Autodesk Inventor part; units mm, degrees
ref_plane "YZ Plane" through (0, 0, 0) normal (1, 0, 0) x (0, 1, 0)
ref_plane "XZ Plane" through (0, 0, 0) normal (0, 1, 0) x (-1, 0, 0)
ref_plane "XY Plane" through (0, 0, 0) normal (0, 0, 1) x (1, 0, 0)
sketch "スケッチ1" plane through (0, 0, 0) normal (0, 0, 1) x (1, 0, 0)
  line L0 (-12.5, -12.5) -> (12.5, -12.5) construction
  line L1 (12.5, -12.5) -> (12.5, 12.5) construction
  line L2 (12.5, 12.5) -> (-12.5, 12.5) construction
  line L3 (-12.5, 12.5) -> (-12.5, -12.5) construction
  line L4 (-12.5, -12.5) -> (12.5, 12.5) construction
  line L5 (12.5, -12.5) -> (-12.5, 12.5) construction
  line L6 (-8.1, 12.5) -> (-12.5, 12.5)
  line L7 (-12.5, 12.5) -> (-12.5, 8.1)
  line L8 (8.1, 12.5) -> (12.5, 12.5)
  line L9 (12.5, 12.5) -> (12.5, 8.1)
  line L10 (-12.5, -8.1) -> (-12.5, -12.5)
  line L11 (-12.5, -12.5) -> (-8.1, -12.5)
  line L12 (8.1, -12.5) -> (12.5, -12.5)
  line L13 (12.5, -12.5) -> (12.5, -8.1)
  line L14 (-6, 12.5) -> (-6, 14.5)
  line L15 (-6, 14.5) -> (6, 14.5)
  line L16 (6, 14.5) -> (6, 12.5)
  arc A0 (-8.1, 12.5) -> (-6, 12.5) centre (-7.05, 12.5) ccw
  arc A1 (6, 12.5) -> (8.1, 12.5) centre (7.05, 12.5) ccw
  line L17 (0, 12.5) -> (0, 0) construction
  line L18 (0, 0) -> (12.5, 0) construction
  line L19 (-12.5, 6) -> (-14.5, 6) construction
  line L20 (-14.5, 6) -> (-14.5, -6) construction
  line L21 (-14.5, -6) -> (-12.5, -6) construction
  arc A2 (-12.5, 6) -> (-12.5, 8.1) centre (-12.5, 7.05) ccw
  arc A3 (-12.5, -8.1) -> (-12.5, -6) centre (-12.5, -7.05) ccw construction
  line L22 (-6, -12.5) -> (-6, -14.5)
  line L23 (-6, -14.5) -> (6, -14.5)
  line L24 (6, -14.5) -> (6, -12.5)
  arc A4 (-6, -12.5) -> (-8.1, -12.5) centre (-7.05, -12.5) ccw
  arc A5 (8.1, -12.5) -> (6, -12.5) centre (7.05, -12.5) ccw
  line L25 (12.5, 6) -> (14.5, 6) construction
  line L26 (14.5, 6) -> (14.5, -6) construction
  line L27 (14.5, -6) -> (12.5, -6) construction
  arc A6 (12.5, 8.1) -> (12.5, 6) centre (12.5, 7.05) ccw construction
  arc A7 (12.5, -6) -> (12.5, -8.1) centre (12.5, -7.05) ccw construction
  line L28 (-9.05, 12.5) -> (-5.95, 12.5) construction
  line L29 (-5.95, 12.5) -> (-5.95, 9.5) construction
  line L30 (-5.95, 9.5) -> (-9.05, 9.5) construction
  line L31 (-9.05, 9.5) -> (-9.05, 12.5) construction
  line L32 (-12.5, 9.05) -> (-9.5, 9.05) construction
  line L33 (-9.5, 9.05) -> (-9.5, 5.95) construction
  line L34 (-9.5, 5.95) -> (-12.5, 5.95) construction
  line L35 (-12.5, 5.95) -> (-12.5, 9.05) construction
  line L36 (-6.7322, 8.5) -> (6.7322, 8.5)
  line L37 (6.7322, 8.5) -> (0, 1.7678)
  line L38 (0, 1.7678) -> (-6.7322, 8.5)
  line L39 (-8.5, 6.7322) -> (-8.5, -6.7322)
  line L40 (-8.5, -6.7322) -> (-1.7678, 0)
  line L41 (-1.7678, 0) -> (-8.5, 6.7322)
  line L42 (-6.7322, -8.5) -> (6.7322, -8.5)
  line L43 (6.7322, -8.5) -> (0, -1.7678)
  line L44 (0, -1.7678) -> (-6.7322, -8.5)
  line L45 (8.5, 6.7322) -> (8.5, -6.7322)
  line L46 (8.5, -6.7322) -> (1.7678, 0)
  line L47 (1.7678, 0) -> (8.5, 6.7322)
  line L48 (-7.5, 12.5) -> (-7.5, 9.5) construction
  line L49 (-9.5, 7.5) -> (-12.5, 7.5) construction
  line L50 (-12.5, -12.5) -> (-12.5, 12.5)
  line L51 (12.5, -12.5) -> (12.5, 12.5)
  dimension "d0" = 25
  dimension "d1" = 1.05
  dimension "d2" = 2
  dimension "d3" = 6.5
  dimension "d4" = 3.1
  dimension "d6" = 3
  dimension "d8" = 3
  dimension "d9" = 2.5
  dimension "d10" = 2.5
  dimension "d11" = 2.5
  dimension "d12" = 2.5
  dimension "d13" = 4
  dimension "d17" = 5
  dimension "d18" = 5
  dimension "d31" = 25
extrude "押し出し1" add sketch "スケッチ1" along normal blind 2.5
mirror "ミラー1" about plane through (0, 0, 0) normal (0, 0, -1) of "押し出し1"
sketch "スケッチ2" plane through (-12.5, -12.5, 2.5) normal (0, -1, 0) x (1, 0, 0)
  line L0 (0, -5) -> (0, 0)
  line L1 (6.5, 0) -> (18.5, 0) construction
  line L2 (12.5, 0) -> (12.5, -5) construction
  point P0 (12.5, -2.5)
  point P1 (2.7, -2.5)
  point P2 (22.3, -2.5)
  point P3 (0, -2.5)
  dimension "d19" = 2.7
hole "穴1" at (-9.8, -12.5, 0) at (9.8, -12.5, 0) direction (0, 1, 0) diameter 2.459 depth 8.8
pattern_circular "円形状パターン1" count 2 over 360 about axis through (0, 0, -10) along (0, 0, 1) of "穴1"
fillet "フィレット1" radius 2 12 edges at (8.5, 6.7322, 0) (8.5, -6.7322, 0) (6.7322, -8.5, 0) (0, 1.7678, 0) (-1.7678, 0, 0) (-6.7322, -8.5, 0) (-8.5, -6.7322, 0) (6.7322, 8.5, 0) (-8.5, 6.7322, 0) (-6.7322, 8.5, 0) (0, -1.7678, 0) (1.7678, 0, 0)
equation "\"d8\" = d6"
equation "\"d10\" = d9"
equation "\"d11\" = d10"
equation "\"d12\" = d11"
equation "\"d18\" = d17"
properties part number "Head_horizontal_frame_02" material "アセタール樹脂、黒"
Here's how the part is built. I have some questions about the finished solid (model axes, mm). A direction names the side the tool comes from. Round coordinates to 2 decimals unless told otherwise and drop trailing zeros. Write each loop counter-clockwise with the first axis right and the second up, starting at its lowest first coordinate (ties: lowest second). Pieces come first, ordered by that corner, then holes.
1. I need wall thicknesses on L1, parallel to X at y = 8.75, z = 0; L2, parallel to X at y = -7, z = 0; L3, parallel to Z at x = 9.8, y = -6. Which ranges of each line are inside material? Lowest first, please.
2. Will these pins go through, and if not, where does the flat tip stop? pin 1 Ø3 at (x, z) = (-9.8, 0) entering from +Y; pin 2 Ø2 at (x, z) = (-9.8, 0) entering from -Y; pin 3 Ø0.6 at (y, z) = (14, -0.5) entering from -X.
3. Suppose I cut it at D-D (z = 0). State how many separate pieces and enclosed holes the cut face has, and give its area (3 significant figures).
4. Suppose I cut it at A-A (y = -4.25). List the corners of the cut face in (x, z) for me.
5. For faces 1 (the flat face through (6, 14, 0)), 2 (the flat face through (0, -8.5, 0)), 3 (the flat face through (11.2, -12.5, 0)), 4 (the cylindrical face through (9.052, 8.038, 0.976)), which set-ups out of +Z, -Z, +X, -X, +Y, -Y let a thin tool reach every point of the face, with its end or its side?
6. Suppose I cut it at C-C (y = -0.25). List the corners of the cut face in (x, z) for me.
7. If we mould it in two halves opening along Y, with no side actions, what happens to faces 5 (the flat face through (0, -14.5, 0)), 6 (the flat face through (11.2, 12.5, 0)), 7 (the flat face through (2.38, 4.15, -0.04)), 8 (the flat face through (0, 0, -2.5))? For each: released by +Y, released by -Y, zero draft, split by the parting line, or undercut.
8. Suppose I cut it at B-B (x = 4.5). List the corners of the cut face in (y, z) for me.
Answer sheet:
1. L1: x = -12.5 to -11.03, -8.57 to 8.57, 11.03 to 12.5
1. L2: x = -12.5 to -11.03, -8.57 to -3.84, 3.84 to 8.57, 11.03 to 12.5
1. L3: z = -2.5 to -1.23, 1.23 to 2.5
2. pin 1: stops at y = 12.5
2. pin 2: stops at y = -3.7
2. pin 3: stops at x = -6
3. separate pieces: 1
3. enclosed holes: 4
3. area: 441 mm2
4. outline: (-12.5, -2.5) - (-2.48, -2.5) - (-2.48, 2.5) - (-12.5, 2.5) - close; (2.48, -2.5) - (12.5, -2.5) - (12.5, 2.5) - (2.48, 2.5) - close; hole circle Ø2.46 at (-9.8, 0); hole circle Ø2.46 at (9.8, 0)
5. face 1: +Z, -Z, +X, +Y
5. face 2: +Z, -Z
5. face 3: +Z, -Z, +X, -Y
5. face 4: +Y
6. outline: (-12.5, -2.5) - (-8.5, -2.5) - (-8.5, 2.5) - (-12.5, 2.5) - close; (-2.61, -2.5) - (2.61, -2.5) - (2.61, 2.5) - (-2.61, 2.5) - close; (8.5, -2.5) - (12.5, -2.5) - (12.5, 2.5) - (8.5, 2.5) - close
7. face 5: released by -Y
7. face 6: released by +Y
7. face 7: undercut
7. face 8: zero draft
8. outline: (-14.5, -2.5) - (-2.73, -2.5) - (-2.73, 2.5) - (-14.5, 2.5) - close; (2.73, -2.5) - (14.5, -2.5) - (14.5, 2.5) - (2.73, 2.5) - close
